Part model, mm, in its own coordinate system. A direction names the side the tool comes from. Round coordinates to 2 decimals unless told otherwise and drop trailing zeros. Write each loop counter-clockwise with the first axis right and the second up, starting at its lowest first coordinate (ties: lowest second). Pieces come first, ordered by that corner, then holes.
```python
from build123d import *

# Parameters (mm, degrees)
F0_W      = 110
F0_H      = 60
F0_W_2    = 48.96
F0_H_2    = 36.72
F1_DEPTH  = 1.2
F2_R      = 7.2
F2_R_2    = 6
F3_DEPTH  = 5
F4_DEPTH  = 5
F5_R      = 1.5
F6_DEPTH  = 25
F7_R      = 5
F8_R      = 3
F8_R_2    = 1.4
F9_DEPTH  = 21
F10_R     = 3
F10_R_2   = 1.4
F11_DEPTH = 4
F12_W     = 75
F12_H     = 1.6
F12_W_2   = 1.6
F12_H_2   = 30
F13_DEPTH = 3.2


with BuildPart() as f1:
    # F0 (on Top) → F1 (new body)
    with BuildSketch(Plane.XY):
        with Locations((2.58, 0)):
            Rectangle(F0_W, F0_H)
        with Locations((2.58, 0)):
            Rectangle(F0_W_2, F0_H_2, mode=Mode.SUBTRACT)
    extrude(amount=F1_DEPTH)

    # F2 (on face) → F3 (join)
    with BuildSketch(Plane.XY.offset(1.2)):
        with Locations((46.58, 16)):
            Circle(F2_R)
        with Locations((46.58, 16)):
            Circle(F2_R_2, mode=Mode.SUBTRACT)
    extrude(amount=F3_DEPTH)

    # F2 (on face) → F4 (join)
    with BuildSketch(Plane.XY.offset(1.2)):
        with Locations((46.58, 16)):
            Circle(F2_R)
        with Locations((46.58, 16)):
            Circle(F2_R_2, mode=Mode.SUBTRACT)
    extrude(amount=F4_DEPTH)

    # F5 (on face) → F6 (cut)
    with BuildSketch(Plane.XY.offset(1.2)):
        with Locations((46.58, 16)):
            Circle(F5_R)
    extrude(amount=-F6_DEPTH, mode=Mode.SUBTRACT)

    # F7
    f7_edges = [f1.edges().sort_by_distance(p)[0] for p in [
        (57.58, 30, 0.6),
        (-52.42, 30, 0.6),
        (-52.42, -30, 0.6),
        (57.58, -30, 0.6),
    ]]
    fillet(f7_edges, radius=F7_R)

    # F8 (on face) → F9 (join)
    with BuildSketch(Plane.XY.offset(1.2)):
        with Locations((52.58, 25)):
            Circle(F8_R)
        with Locations((52.58, 25)):
            Circle(F8_R_2, mode=Mode.SUBTRACT)
        with Locations((52.58, -25)):
            Circle(F8_R)
        with Locations((52.58, -25)):
            Circle(F8_R_2, mode=Mode.SUBTRACT)
        with Locations((-47.42, -25)):
            Circle(F8_R)
        with Locations((-47.42, -25)):
            Circle(F8_R_2, mode=Mode.SUBTRACT)
        with Locations((-47.42, 25)):
            Circle(F8_R)
        with Locations((-47.42, 25)):
            Circle(F8_R_2, mode=Mode.SUBTRACT)
    extrude(amount=F9_DEPTH)

    # F10 (on face) → F11 (join)
    with BuildSketch(Plane.XY.offset(1.2)):
        with Locations((34.16, -18.25)):
            Circle(F10_R)
        with Locations((34.16, -18.25)):
            Circle(F10_R_2, mode=Mode.SUBTRACT)
        with Locations((-34.16, -18.25)):
            Circle(F10_R)
        with Locations((-34.16, -18.25)):
            Circle(F10_R_2, mode=Mode.SUBTRACT)
        with Locations((34.16, 18.25)):
            Circle(F10_R)
        with Locations((34.16, 18.25)):
            Circle(F10_R_2, mode=Mode.SUBTRACT)
        with Locations((-34.16, 18.25)):
            Circle(F10_R)
        with Locations((-34.16, 18.25)):
            Circle(F10_R_2, mode=Mode.SUBTRACT)
    extrude(amount=F11_DEPTH)

    # F12 (on face) → F13 (join)
    with BuildSketch(Plane.XY.offset(1.2)):
        with Locations((3.115936, -27.6)):
            Rectangle(F12_W, F12_H)
        with Locations((3.115936, 27.6)):
            Rectangle(F12_W, F12_H)
        with Locations((-50.02, 0)):
            Rectangle(F12_W_2, F12_H_2)
        with Locations((55.18, 0)):
            Rectangle(F12_W_2, F12_H_2)
    extrude(amount=F13_DEPTH)


solid = f1.part
```
Q1. Cut at B-B on z = 3. State how many separate pieces and enclosed holes the cut face has, plus the area to 3 significant figures.
Values follow:
separate pieces: 13
enclosed holes: 9
area: 563 mm2
Q2. Cut at D-D on y = 5. Write the cut outline in (x, z).
Values follow:
outline: (-52.42, 0) - (-21.9, 0) - (-21.9, 1.2) - (-49.22, 1.2) - (-49.22, 4.4) - (-50.82, 4.4) - (-50.82, 1.2) - (-52.42, 1.2) - close; (27.06, 0) - (57.58, 0) - (57.58, 1.2) - (55.98, 1.2) - (55.98, 4.4) - (54.38, 4.4) - (54.38, 1.2) - (27.06, 1.2) - close
Q3. Wall check: L1, parallel to Y at x = 52.58, z = 14.5; L2, parallel to Y at x = 46.58, z = 0.9; L3, parallel to X at y = 19, z = 3.75. Give the ranges that are in metal, low to high.
Values follow:
L1: y = -28 to -26.4, -23.6 to -22, 22 to 23.6, 26.4 to 28
L2: y = -30 to 14.5, 17.5 to 30
L3: x = -37.06 to -35.34, -32.98 to -31.26, 31.26 to 32.98, 35.34 to 37.06, 40.03 to 41.38, 51.78 to 53.13
Q4. Mould opens along Y. For faces 5 (the cylindrical face through (31.8, 16.4, 3.2)), 6 (the flat face through (54, -26, 22.2)), 7 (the flat face through (3, 28.4, 3)) say: +Y half, -Y half, draft (parallel to the pull), parting line (faces both ways), or undercut.
Values follow:
face 5: undercut
face 6: draft
face 7: +Y half
Q5. Cut at A-A on z = 19.25. Write the cut outline in (x, y), plus the area to 3 significant figures.
Values follow:
outline: circle Ø6 at (-47.42, -25); circle Ø6 at (-47.42, 25); circle Ø6 at (52.58, -25); circle Ø6 at (52.58, 25); hole circle Ø2.8 at (-47.42, -25); hole circle Ø2.8 at (-47.42, 25); hole circle Ø2.8 at (52.58, -25); hole circle Ø2.8 at (52.58, 25)
area: 88.5 mm2
Q6. Cut at C-C on x = 46.58. Write the cut outline in (y, z).
Values follow:
outline: (-30, 0) - (14.5, 0) - (14.5, 1.2) - (10, 1.2) - (10, 6.2) - (8.8, 6.2) - (8.8, 1.2) - (-30, 1.2) - close; (17.5, 0) - (30, 0) - (30, 1.2) - (23.2, 1.2) - (23.2, 6.2) - (22, 6.2) - (22, 1.2) - (17.5, 1.2) - close
Q7. Drop flat-ended pins along their axis: pin 1 (1.7 mm diameter, centred on x = 34.16, y = -18.25, fed in from +Z); pin 2 (13 mm diameter, centred on x = 44, y = 16.5, fed in from +Z); pin 3 (3 mm diameter, centred on y = 8, z = 6, fed in from +X). Give the stop position or say it passes through.
Values follow:
pin 1: stops at z = 1.2
pin 2: stops at z = 6.2
pin 3: stops at x = 49.68
Q8. Which spindle directions (+Z, -Z, +X, -X, +Y, -Y) get a long thin tool onto all of the face, cutting with end or side? Do faces 1 (the flat face through (-34, -18, 1.2)), 2 (the flat face through (55.98, 0, 3)), 3 (the flat face through (-50.82, 0, 3)), 4 (the cylindrical face through (56.08, 28.57, 0.61)). Say none if no direction does.
Values follow:
face 1: +Z
face 2: +Z, +X, +Y, -Y
face 3: +Z, -X, +Y, -Y
face 4: +Z, -Z, +X, +Y
